Read the model definition and answer for the solid it produces. Units are mm, in the model's axes. A direction names the side the tool comes from. Coordinates: 2 decimals unless noted, no trailing zeros. Write each loop counter-clockwise with the first axis right and the second up, starting at its lowest first coordinate (ties: lowest second). Pieces come first, ordered by that corner, then holes. Notation, with made-up numbers: (11.25, 23) -> (55.25, 23) arc R23 ccw to (55.25, 39) -> close; hole circle Ø8 at (28, -35.75). An arc over 180 degrees is marked (long way). Return JSON: item names as keys, results as strings.
Solid Edge part; units mm, degrees
sketch "Sketch1" plane through (0, 0, 0) normal (0, 0, 1) x (1, 0, 0)
  circle A0 centre (0, 0) radius 3.5
extrude "Protrusion1" add sketch "Sketch1" along normal blind 4
sketch "Sketch2" plane through (0, 0, 0) normal (0, 0, -1) x (1, 0, 0)
  line L0 (0.85, 1.4722) -> (1.7, 0)
  line L1 (1.7, 0) -> (0.85, -1.4722)
  line L2 (0.85, -1.4722) -> (-0.85, -1.4722)
  line L3 (-0.85, -1.4722) -> (-1.7, 0)
  line L4 (-1.7, 0) -> (-0.85, 1.4722)
  line L5 (-0.85, 1.4722) -> (0.85, 1.4722)
extrude "ExtrudedCutout_1" cut sketch "Sketch2" against normal blind 2.4
sketch "Sketch3" plane through (0, 0, 4) normal (0, 0, 1) x (-1, 0, 0)
  circle A0 centre (0, 0) radius 2
extrude "ExtrudedProtrusion_2" add sketch "Sketch3" along normal blind 20
cosmetic_thread "Thread_1" thread depth 20
1. Consider L1, parallel to Z at x = -1.5, y = -1.75; L2, parallel to Z at x = 0.5, y = -0.5; L3, parallel to Y at x = 0.75, z = 1.75. Determine where each line is inside the solid, lowest interval first.
Taken from the geometry:
{"L1": "z = 0 to 4", "L2": "z = 2.4 to 24", "L3": "y = -3.42 to -1.47, 1.47 to 3.42"}
2. The part is cut by section D-D (y = 1.75). Determine the outline of the cut face in (x, z).
Taken from the geometry:
{"outline": "(-3.03, 0) -> (3.03, 0) -> (3.03, 4) -> (0.97, 4) -> (0.97, 24) -> (-0.97, 24) -> (-0.97, 4) -> (-3.03, 4) -> close"}
3. For a pull along X with two mould halves and no side action, classify faces 1 (the face through (3.233, 1.341, 1.972)), 2 (the face through (-1.269, 0.746, 1.183)), 3 (the face through (2, -2, 4)) as +X half, -X half, draft (parallel to the pull), parting line (faces both ways), or undercut.
Taken from the geometry:
{"face 1": "parting line", "face 2": "undercut", "face 3": "draft"}
4. A tool of negligible diameter and unlimited length cuts with its end or side. For faces 4 (the face through (0, -2, 14)), 5 (the face through (-1.28, -0.73, 1.18)), 6 (the face through (0, -2, 0)), from which of +Z, -Z, +X, -X, +Y, -Y can it reach the whole face along a straight path? Write none if from no direction.
Taken from the geometry:
{"face 4": "+Z", "face 5": "-Z", "face 6": "-Z, +X, -X, +Y, -Y"}
5. The part is cut by section B-B (y = 0.25). Determine the outline of the cut face in (x, z).
Taken from the geometry:
{"outline": "(-3.49, 0) -> (-1.56, 0) -> (-1.56, 2.4) -> (1.56, 2.4) -> (1.56, 0) -> (3.49, 0) -> (3.49, 4) -> (1.98, 4) -> (1.98, 24) -> (-1.98, 24) -> (-1.98, 4) -> (-3.49, 4) -> close"}
6. The part is cut by section C-C (z = 5.75). Determine the outline of the cut face in (x, y).
Taken from the geometry:
{"outline": "circle Ø4 at (0, 0)"}
7. Flat-ended cylindrical pins translate along their axes: pin 1 Ø0.9 at (x, y) = (-0.5, 0) entering from -Z; pin 2 Ø3 at (x, z) = (1.5, 9) entering from -Y; pin 3 Ø4 at (x, z) = (2.5, 2.5) entering from +Y. Find the tip coordinate at first contact, or state that the pin passes through.
Taken from the geometry:
{"pin 1": "stops at z = 2.4", "pin 2": "stops at y = -2", "pin 3": "stops at y = 3.46"}
8. The part is cut by section A-A (x = 0). Determine the outline of the cut face in (y, z), then the cut area to 3 significant figures.
Taken from the geometry:
{"outline": "(-3.5, 0) -> (-1.47, 0) -> (-1.47, 2.4) -> (1.47, 2.4) -> (1.47, 0) -> (3.5, 0) -> (3.5, 4) -> (2, 4) -> (2, 24) -> (-2, 24) -> (-2, 4) -> (-3.5, 4) -> close", "area": "101 mm2"}
